Can you work these out from the model? Positions are in its coordinate system, mm. Face numbers are marked on the shaded views. A direction names the side the tool comes from. Round coordinates to 2 decimals unless told otherwise and drop trailing zeros. Write each loop counter-clockwise with the first axis right and the second up, starting at its lowest first coordinate (ties: lowest second). Pieces come first, ordered by that corner, then holes. Notation, with made-up numbers: M 81.25,22 L 140.25,22 A24 cw 140.25,34 Z; hole C 70,17.5 d10. An arc over 180 degrees is marked long. Answer as a JSON object with one key per item and string values. Group by question number.
1) Suppose I cut it at A-A, the plane z = 0. Write out the boundary of the cut face in (x, y).
2) Suppose I cut it at D-D, the plane y = 63. Write out the boundary of the cut face in (x, z).
3) On a 3-axis mill with a long thin cutter (end or side, diameter ignored), from which of +Z, -Z, +X, -X, +Y, -Y can I reach the whole of each face in a straight line? I mean the marked faces 4, 5 and 6. Say none if no direction works.
4) Suppose I cut it at B-B, the plane y = 118.1. Write out the boundary of the cut face in (x, z).
5) Suppose I cut it at C-C, the plane x = 20. Write out the boundary of the cut face in (y, z).
6) I'm going to push flat-ended pins straight in: pin 1 Ø12 at (y, z) = (47, 24) entering from -X; pin 2 Ø18 at (x, y) = (11.5, 109) entering from +Z; pin 3 Ø17 at (y, z) = (127, 5.5) entering from -X; pin 4 Ø6.5 at (y, z) = (118.1, 0) entering from -X. Where does each tip first touch, or does it pass through?
7) If we mould it in two halves opening along Y, with no side actions, what happens to the marked faces 1, 2 and 3? For each: +Y half, -Y half, draft (parallel to the pull), parting line (faces both ways), or undercut.
8) Please list where these lines run through material, in increasing order: L1, parallel to Y at x = 29.25, z = 0; L2, parallel to Y at x = -27.5, z = 24; L3, parallel to Z at x = 32, y = 118. Write a range as [from, to].
from build123d import *

# Parameters (mm, degrees)
BOSS_EXTRUDE1_DEPTH = 5
BOSS_EXTRUDE2_DEPTH = 80
SKETCH4_R           = 4.1
BOSS_EXTRUDE3_DEPTH = 8
BOSS_EXTRUDE4_DEPTH = 3


with BuildPart() as part:
    # Sketch2 → Boss-Extrude1 (new body)
    with BuildSketch(Plane(origin=(0, 0, 0), x_dir=(1, 0, 0), z_dir=(0, 1, 0))):
        with BuildLine():
            Line((-30, -35), (30, -35))
            ThreePointArc((30, -35), (33.535533906, -33.535533906), (35, -30))
            Line((35, -30), (35, 30))
            ThreePointArc((35, 30), (33.535533906, 33.535533906), (30, 35))
            Line((30, 35), (-30, 35))
            ThreePointArc((-30, 35), (-33.535533906, 33.535533906), (-35, 30))
            Line((-35, 30), (-35, -30))
            ThreePointArc((-35, -30), (-33.535533906, -33.535533906), (-30, -35))
        make_face()
    boss_extrude1 = extrude(amount=BOSS_EXTRUDE1_DEPTH)

    # Sketch3 → Boss-Extrude2 (add)
    with BuildSketch(Plane(origin=(0, 5, 0), x_dir=(1, 0, 0), z_dir=(0, 1, 0))):
        Polygon((-2.5, 2.5), (-2.5, 35), (2.5, 35), (2.5, 2.5), (35, 2.5), (35, -2.5), (2.5, -2.5), (2.5, -35), (-2.5, -35), (-2.5, -2.5), (-35, -2.5), (-35, 2.5), align=None)
    extrude(amount=BOSS_EXTRUDE2_DEPTH)

    # Mirror1: Boss-Extrude1 across plane
    add(boss_extrude1.mirror(Plane.ZX.offset(45)))

    # Sketch4 → Boss-Extrude3 (add)
    with BuildSketch(Plane(origin=(35, 0, 0), x_dir=(0, 0, -1), z_dir=(1, 0, 0))):
        with BuildLine():
            Line((-28.25, 90), (28.25, 90))
            Line((28.25, 90), (28.25, 126.2))
            ThreePointArc((28.25, 126.2), (22.392135624, 140.342135624), (8.25, 146.2))
            Line((8.25, 146.2), (-8.25, 146.2))
            ThreePointArc((-8.25, 146.2), (-22.392135624, 140.342135624), (-28.25, 126.2))
            Line((-28.25, 126.2), (-28.25, 90))
        make_face()
        with Locations((0, 118.1)):
            Circle(SKETCH4_R, mode=Mode.SUBTRACT)
    extrude(amount=-BOSS_EXTRUDE3_DEPTH)

    # Sketch5 → Boss-Extrude4 (add)
    with BuildSketch(Plane.XY.offset(28.25)):
        Polygon((35, 90), (-30, 90), (27, 126.2), (35, 126.2), align=None)
    boss_extrude4 = extrude(amount=-BOSS_EXTRUDE4_DEPTH)

    # Mirror2: Boss-Extrude4 across plane
    add(boss_extrude4.mirror(Plane(origin=(0, 0, 0), x_dir=(1, 0, 0), z_dir=(0, 0, -1))))


solid = part.part
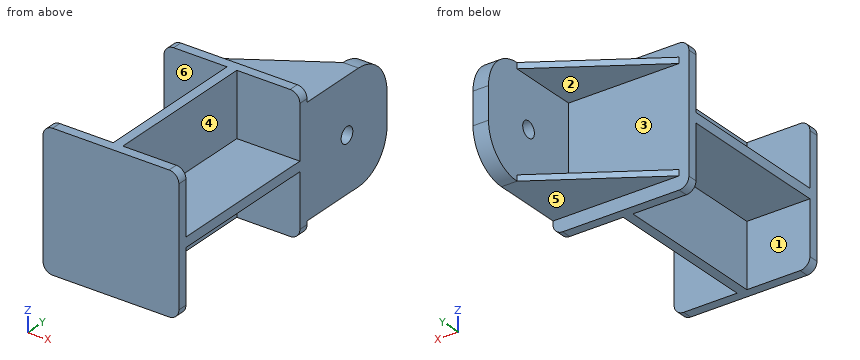
Results:
{
 "1": {"outline": "M -35,0 L 35,0 L 35,114 L 27,114 L 27,90 L -35,90 Z; M 27,122.2 L 35,122.2 L 35,146.2 L 27,146.2 Z"},
 "2": {"outline": "M -35,-2.5 L -2.5,-2.5 L -2.5,-35 L 2.5,-35 L 2.5,-2.5 L 35,-2.5 L 35,2.5 L 2.5,2.5 L 2.5,35 L -2.5,35 L -2.5,2.5 L -35,2.5 Z"},
 "3": {"face 4": "+Z, +X", "face 5": "-Z, +X, -X, +Y", "face 6": "+Z, -X"},
 "4": {"outline": "M 14.25,-28.25 L 35,-28.25 L 35,-4.1 L 27,-4.1 L 27,-25.25 L 14.25,-25.25 Z; M 14.25,25.25 L 27,25.25 L 27,4.1 L 35,4.1 L 35,28.25 L 14.25,28.25 Z"},
 "5": {"outline": "M 0,-35 L 5,-35 L 5,-2.5 L 85,-2.5 L 85,-35 L 90,-35 L 90,-28.25 L 121.75,-28.25 L 121.75,-25.25 L 90,-25.25 L 90,25.25 L 121.75,25.25 L 121.75,28.25 L 90,28.25 L 90,35 L 85,35 L 85,2.5 L 5,2.5 L 5,35 L 0,35 Z"},
 "6": {"pin 1": "x = -2.5", "pin 2": "z = 28.25", "pin 3": "x = 27", "pin 4": "through"},
 "7": {"face 1": "undercut", "face 2": "draft", "face 3": "+Y half"},
 "8": {"L1": "[0, 114], [122.2, 146.2]", "L2": "[0, 5], [85, 90]", "L3": "[-28.25, -4.1], [4.1, 28.25]"}
}
